Geometry check sheet. Reference: the model listing, model coordinates, mm. Give positions to 0.01 mm unless a question says otherwise; leave off trailing zeros. Order: outer loops, then holes, each group sorted by start corner. A loop starts at its lowest first (then second) coordinate and runs counter-clockwise, first axis right, second up. Notation, with made-up numbers: M -38,-10.5 L -25,-10.5 A35 ccw -25,25.5 Z; hole C -3.75,59.5 d10. An arc over 180 degrees is marked long. Put each result on its own line as item: value. Start each with the question number.
Q1. Material ranges on L1, parallel to X at y = 62.5, z = 4.3; L2, parallel to X at y = 65, z = 4.6; L3, parallel to Y at x = 50.5, z = 3.15, recorded low to high.
Q2. Section check A-A on y = 61. Record the cut outline in (x, z).
Q3. Section check D-D on z = 3.3. State how many separate pieces and enclosed holes the cut face has, then the cut area to 3 significant figures.
Q4. Section check B-B on x = -9. Record the cut outline in (y, z), then the cut area to 3 significant figures.
Q5. Go/stop test with a flat-tipped pin: pin 1 (3 mm diameter, centred on x = 34, y = 0, fed in from -Z). Record where the tip stops, or that it passes through.
Q6. Section check C-C on y = 0. Record the cut outline in (x, z).
```python
from build123d import *

# Parameters (mm, degrees)
SKETCH_1_W          = 151.1
SKETCH_1_H          = 60
SKETCH_1_R          = 3
SKETCH_1_R_2        = 1.6
SKETCH_1_W_2        = 3.1
SKETCH_1_H_2        = 10
EXTRUDE_1_DEPTH     = 5
SKETCH_2_R          = 1.55
SKETCH_2_W          = 25.45
SKETCH_2_H          = 18
CUT_EXTRUDE_1_DEPTH = 82.442019253
FILLET_1_R          = 3
SKETCH_3_W          = 151.1
SKETCH_3_H          = 60
SKETCH_3_W_2        = 6
SKETCH_3_H_2        = 6
SKETCH_3_W_3        = 33.1
SKETCH_3_H_3        = 54
EXTRUDE_2_DEPTH     = 5
SKETCH_4_W          = 34
SKETCH_4_H          = 46
SKETCH_4_W_2        = 30
CUT_EXTRUDE_2_DEPTH = 118.612935088
FILLET_2_R          = 5
CHAMFER_1_SIZE      = 8


with BuildPart() as part:
    # 草图1 → 凸台-拉伸1 (new body)
    with BuildSketch(Plane.XY):
        Rectangle(SKETCH_1_W, SKETCH_1_H)
        Circle(SKETCH_1_R, mode=Mode.SUBTRACT)
        with Locations((34, 0)):
            Circle(SKETCH_1_R_2, mode=Mode.SUBTRACT)
        with Locations((-34, 0)):
            Circle(SKETCH_1_R_2, mode=Mode.SUBTRACT)
        with Locations((34, -20)):
            Rectangle(SKETCH_1_W_2, SKETCH_1_H_2, mode=Mode.SUBTRACT)
        with Locations((-34, 20)):
            Rectangle(SKETCH_1_W_2, SKETCH_1_H_2, mode=Mode.SUBTRACT)
        with Locations((-34, -20)):
            Rectangle(SKETCH_1_W_2, SKETCH_1_H_2, mode=Mode.SUBTRACT)
        with Locations((34, 20)):
            Rectangle(SKETCH_1_W_2, SKETCH_1_H_2, mode=Mode.SUBTRACT)
    extrude(amount=EXTRUDE_1_DEPTH)

    # 草图2 → 切除-拉伸1 (cut, through all)
    with BuildSketch(Plane.XY.offset(5)):
        with Locations((-34, 25)):
            Circle(SKETCH_2_R)
        with Locations((-34, 15)):
            Circle(SKETCH_2_R)
        with Locations((34, 25)):
            Circle(SKETCH_2_R)
        with Locations((34, 15)):
            Circle(SKETCH_2_R)
        with Locations((34, -15)):
            Circle(SKETCH_2_R)
        with Locations((34, -25)):
            Circle(SKETCH_2_R)
        with Locations((-34, -15)):
            Circle(SKETCH_2_R)
        with Locations((-34, -25)):
            Circle(SKETCH_2_R)
        with Locations((-15.725, 13)):
            Rectangle(SKETCH_2_W, SKETCH_2_H)
        with Locations((15.725, 13)):
            Rectangle(SKETCH_2_W, SKETCH_2_H)
        with Locations((-15.725, -13)):
            Rectangle(SKETCH_2_W, SKETCH_2_H)
        with Locations((15.725, -13)):
            Rectangle(SKETCH_2_W, SKETCH_2_H)
    extrude(amount=-CUT_EXTRUDE_1_DEPTH, mode=Mode.SUBTRACT)

    # 圆角1
    fillet_1_edges = [part.edges().sort_by_distance(p)[0] for p in [
        (28.45, 4, 2.5),
        (3, 4, 2.5),
        (3, 22, 2.5),
        (28.45, 22, 2.5),
        (-28.45, -22, 2.5),
        (-28.45, -4, 2.5),
        (-3, -4, 2.5),
        (-3, -22, 2.5),
        (28.45, -22, 2.5),
        (3, -22, 2.5),
        (3, -4, 2.5),
        (28.45, -4, 2.5),
        (-28.45, 4, 2.5),
        (-28.45, 22, 2.5),
        (-3, 22, 2.5),
        (-3, 4, 2.5),
    ]]
    fillet(fillet_1_edges, radius=FILLET_1_R)

    # 草图3 → 凸台-拉伸2 (add)
    with BuildSketch(Plane.XY.offset(5)):
        with Locations((0, 60)):
            Rectangle(SKETCH_3_W, SKETCH_3_H)
        with Locations((24.55, 48)):
            Rectangle(SKETCH_3_W_2, SKETCH_3_H_2, mode=Mode.SUBTRACT)
        with Locations((-24.55, 61)):
            Rectangle(SKETCH_3_W_2, SKETCH_3_H_2, mode=Mode.SUBTRACT)
        with Locations((-24.55, 48)):
            Rectangle(SKETCH_3_W_2, SKETCH_3_H_2, mode=Mode.SUBTRACT)
        with Locations((24.55, 61)):
            Rectangle(SKETCH_3_W_2, SKETCH_3_H_2, mode=Mode.SUBTRACT)
        with Locations((0, 58)):
            Rectangle(SKETCH_3_W_3, SKETCH_3_H_3, mode=Mode.SUBTRACT)
    extrude(amount=-EXTRUDE_2_DEPTH)

    # 草图4 → 切除-拉伸2 (cut, through all)
    with BuildSketch(Plane.XY.offset(5)):
        with Locations((-52.55, 59)):
            Rectangle(SKETCH_4_W, SKETCH_4_H)
        with Locations((-54.55, 1)):
            Rectangle(SKETCH_4_W_2, SKETCH_4_H)
        with Locations((54.55, 1)):
            Rectangle(SKETCH_4_W_2, SKETCH_4_H)
        with Locations((52.55, 59)):
            Rectangle(SKETCH_4_W, SKETCH_4_H)
    extrude(amount=-CUT_EXTRUDE_2_DEPTH, mode=Mode.SUBTRACT)

    # 圆角2
    fillet_2_edges = [part.edges().sort_by_distance(p)[0] for p in [
        (-16.55, 85, 2.5),
        (16.55, 85, 2.5),
        (16.55, 31, 2.5),
        (-16.55, 31, 2.5),
        (69.55, 82, 2.5),
        (69.55, 36, 2.5),
        (35.55, 36, 2.5),
        (35.55, 82, 2.5),
        (69.55, 24, 2.5),
        (69.55, -22, 2.5),
        (39.55, -22, 2.5),
        (39.55, 24, 2.5),
        (-69.55, -22, 2.5),
        (-69.55, 24, 2.5),
        (-39.55, 24, 2.5),
        (-39.55, -22, 2.5),
        (-69.55, 36, 2.5),
        (-69.55, 82, 2.5),
        (-35.55, 82, 2.5),
        (-35.55, 36, 2.5),
    ]]
    fillet(fillet_2_edges, radius=FILLET_2_R)

    # 倒角1
    chamfer_1_edges = [part.edges().sort_by_distance(p)[0] for p in [
        (-75.55, 90, 2.5),
        (75.55, 90, 2.5),
        (75.55, -30, 2.5),
        (-75.55, -30, 2.5),
    ]]
    chamfer(chamfer_1_edges, length=CHAMFER_1_SIZE)


solid = part.part
```
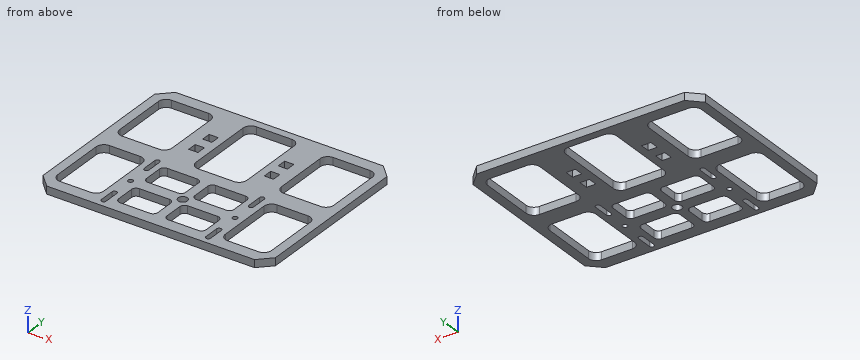
Results found:
1. L1: x = -75.55 to -69.55, -35.55 to -27.55, -21.55 to -16.55, 16.55 to 21.55, 27.55 to 35.55, 69.55 to 75.55
1. L2: x = -75.55 to -69.55, -35.55 to -16.55, 16.55 to 35.55, 69.55 to 75.55
1. L3: y = -30 to -22, 24 to 36, 82 to 90
2. outline: M -75.55,0 L -69.55,0 L -69.55,5 L -75.55,5 Z; M -35.55,0 L -27.55,0 L -27.55,5 L -35.55,5 Z; M -21.55,0 L -16.55,0 L -16.55,5 L -21.55,5 Z; M 16.55,0 L 21.55,0 L 21.55,5 L 16.55,5 Z; M 27.55,0 L 35.55,0 L 35.55,5 L 27.55,5 Z; M 69.55,0 L 75.55,0 L 75.55,5 L 69.55,5 Z
3. separate pieces: 1
3. enclosed holes: 20
3. area: 8,290 mm^2
4. outline: M -30,0 L -22,0 L -22,5 L -30,5 Z; M -4,0 L 4,0 L 4,5 L -4,5 Z; M 22,0 L 31,0 L 31,5 L 22,5 Z; M 85,0 L 90,0 L 90,5 L 85,5 Z
4. area: 150 mm^2
5. pin 1: passes through
6. outline: M -75.55,0 L -69.55,0 L -69.55,5 L -75.55,5 Z; M -39.55,0 L -35.6,0 L -35.6,5 L -39.55,5 Z; M -32.4,0 L -3,0 L -3,5 L -32.4,5 Z; M 3,0 L 32.4,0 L 32.4,5 L 3,5 Z; M 35.6,0 L 39.55,0 L 39.55,5 L 35.6,5 Z; M 69.55,0 L 75.55,0 L 75.55,5 L 69.55,5 Z
